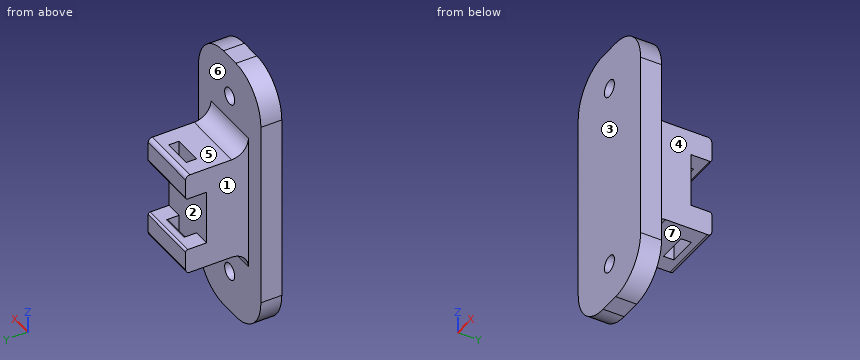
```python
from build123d import *

# Parameters (mm, degrees)
SKETCH1_W           = 25
SKETCH1_H           = 65
BOSS_EXTRUDE1_DEPTH = 5
SKETCH2_R           = 2
CUT_EXTRUDE1_DEPTH  = 6
SKETCH3_W           = 15
SKETCH3_H           = 25
BOSS_EXTRUDE2_DEPTH = 10
SKETCH4_W           = 15
SKETCH4_H           = 6
BOSS_EXTRUDE3_DEPTH = 5
SKETCH5_W           = 7
SKETCH5_H           = 2.5
CUT_EXTRUDE2_DEPTH  = 46
FILLET1_R           = 0.5
FILLET2_R           = 0.5
FILLET3_R           = 1
FILLET4_R           = 10
FILLET5_R           = 4


with BuildPart() as part:
    # Sketch1 → Boss-Extrude1 (new body)
    with BuildSketch(Plane(origin=(0, 0, 0), x_dir=(1, 0, 0), z_dir=(0, 1, 0))):
        with Locations((12.5, 32.5)):
            Rectangle(SKETCH1_W, SKETCH1_H)
    extrude(amount=BOSS_EXTRUDE1_DEPTH)

    # Sketch2 → Cut-Extrude1 (cut, through all)
    with BuildSketch(Plane(origin=(0, 0, 0), x_dir=(1, 0, 0), z_dir=(0, 1, 0))):
        with Locations((12.5, 55)):
            Circle(SKETCH2_R)
        with Locations((12.5, 10)):
            Circle(SKETCH2_R)
    extrude(amount=CUT_EXTRUDE1_DEPTH, mode=Mode.SUBTRACT)

    # Sketch3 → Boss-Extrude2 (add)
    with BuildSketch(Plane(origin=(0, 5, 0), x_dir=(1, 0, 0), z_dir=(0, 1, 0))):
        with Locations((12.5, 32.5)):
            Rectangle(SKETCH3_W, SKETCH3_H)
    extrude(amount=BOSS_EXTRUDE2_DEPTH)

    # Sketch4 → Boss-Extrude3 (add)
    with BuildSketch(Plane(origin=(0, 15, 0), x_dir=(1, 0, 0), z_dir=(0, 1, 0))):
        with Locations((12.5, 42)):
            Rectangle(SKETCH4_W, SKETCH4_H)
        with Locations((12.5, 23)):
            Rectangle(SKETCH4_W, SKETCH4_H)
    extrude(amount=BOSS_EXTRUDE3_DEPTH)

    # Sketch5 → Cut-Extrude2 (cut, through all)
    with BuildSketch(Plane(origin=(0, 0, -45), x_dir=(-1, 0, 0), z_dir=(0, 0, -1))):
        with Locations((-12.5, 16.25)):
            Rectangle(SKETCH5_W, SKETCH5_H)
    extrude(amount=-CUT_EXTRUDE2_DEPTH, mode=Mode.SUBTRACT)

    # Fillet1
    fillet1_edges = [part.edges().sort_by_distance(p)[0] for p in [
        (12.5, 20, -39),
        (12.5, 17.5, -39),
    ]]
    fillet(fillet1_edges, radius=FILLET1_R)

    # Fillet2
    fillet2_edges = [part.edges().sort_by_distance(p)[0] for p in [
        (12.5, 20, -26),
        (12.5, 17.5, -26),
    ]]
    fillet(fillet2_edges, radius=FILLET2_R)

    # Fillet3
    fillet3_edges = [part.edges().sort_by_distance(p)[0] for p in [
        (12.5, 20, -45),
        (12.5, 20, -20),
    ]]
    fillet(fillet3_edges, radius=FILLET3_R)

    # Fillet4
    fillet4_edges = [part.edges().sort_by_distance(p)[0] for p in [
        (0, 2.5, -65),
        (25, 2.5, -65),
        (25, 2.5, 0),
        (0, 2.5, 0),
    ]]
    fillet(fillet4_edges, radius=FILLET4_R)

    # Fillet5
    fillet5_edges = [part.edges().sort_by_distance(p)[0] for p in [
        (12.5, 5, -45),
        (12.5, 5, -20),
    ]]
    fillet(fillet5_edges, radius=FILLET5_R)


solid = part.part
```
Geometry: final body of the model. Coordinates: model frame, mm. Face numbers are marked on the shaded views. A direction names the side the tool comes from. Coordinates: 2 decimals unless noted, no trailing zeros. Order: outer loops, then holes, each group sorted by start corner. A loop starts at its lowest first (then second) coordinate and runs counter-clockwise, first axis right, second up. Notation, with made-up numbers: M -29.75,84.5 L -0.75,84.5 A25 cw -0.75,98.5 Z; hole C 23,-37 d6. An arc over 180 degrees is marked long. Answer as CSV lines item,"result".
Q1. Section D-D on z = -37.5. Return the cut outline in (x, y), and give its area (3 significant figures).
Answers:
outline,"M 0,0 L 25,0 L 25,5 L 20,5 L 20,15 L 5,15 L 5,5 L 0,5 Z"
area,"275 mm^2"
Q2. Section C-C on z = -22.5. Return the cut outline in (x, y), and give its area (4 significant figures).
Answers:
outline,"M 0,0 L 25,0 L 25,5 L 20,5 L 20,20 L 5,20 L 5,5 L 0,5 Z; hole M 9,15 L 16,15 L 16,17.5 L 9,17.5 Z"
area,"332.5 mm^2"
Q3. Section A-A on x = 12.5. Count the separate pieces of the cut face and the enclosed holes in it, and give its area (3 significant figures).
Answers:
separate pieces,"5"
enclosed holes,"0"
area,"571 mm^2"
Q4. Set-up query: the marked faces 4, 5, 6 and 7. Return all of +Z, -Z, +X, -X, +Y, -Y with unobstructed straight access to the full face (end or side cutting, diameter ignored); none if empty.
Answers:
face 4,"+Z, -Z, +X, +Y"
face 5,"+Z, +X, -X, +Y"
face 6,"+Y"
face 7,"-Z, +X, -X, +Y"
Q5. First-contact query: P1, Ø12, axis at y = 14, z = -34, coming from the +X side; P2, Ø5, axis at x = 12.5, z = -10, coming from the +Y side; P3, Ø1.5, axis at y = 17, z = -43.5, coming from the -X side. Flat tips, straight axial feed; report the tip coordinate or a pass-through.
Answers:
P1,"stops at x = 20"
P2,"stops at y = 5"
P3,"stops at x = 5"
Q6. Line query: probe 1 along Z at (x, y) = (12.5, 1.3); probe 2 along Z at (x, y) = (17, 17.75); probe 3 along X at (y, z) = (3.2, -55). Output: solid intervals per line, ascending. Write a range as [from, to].
Answers:
probe 1,"z = [-65, -57], [-53, -12], [-8, 0]"
probe 2,"z = [-45, -39], [-26, -20]"
probe 3,"x = [0, 10.5], [14.5, 25]"
Q7. Draft query along X for the marked faces 1, 2 and 3. Return one class per face: pulls with the +X half, pulls with the -X half, needs draft (parallel to the pull), parting line crosses it, or undercut.
Answers:
face 1,"pulls with the -X half"
face 2,"undercut"
face 3,"needs draft"
Q8. Section B-B on y = 1.5. Return the cut outline in (x, z), and give its area (3 significant figures).
Answers:
outline,"M 0,-55 A10 ccw 10,-65 L 15,-65 A10 ccw 25,-55 L 25,-10 A10 ccw 15,0 L 10,0 A10 ccw 0,-10 Z; hole C 12.5,-55 d4; hole C 12.5,-10 d4"
area,"1,510 mm^2"
